Build history of the part. All positions in model axes, mm. A direction names the side the tool comes from. Give positions to 0.01 mm unless a question says otherwise; leave off trailing zeros. Order: outer loops, then holes, each group sorted by start corner. A loop starts at its lowest first (then second) coordinate and runs counter-clockwise, first axis right, second up. Notation, with made-up numbers: (62.25, -36.75) - (106.25, -36.75) arc R28 ccw to (106.25, -10.75) - close; hole circle Ø1 at (25.5, -10). An arc over 180 degrees is marked (long way). Answer in a Markdown table with one row per item.
```python
from build123d import *

# Parameters (mm, degrees)
BOSS_EXTRUDE1_DEPTH      = 13.97
BOSS_EXTRUDE1_DEPTH_BACK = 2.38125
SKETCH1_W                = 65.5
SKETCH1_H                = 47
SKETCH1_W_2              = 62.5
SKETCH1_H_2              = 44
SKETCH2_W                = 3.58
SKETCH2_H                = 3.58
BOSS_EXTRUDE2_DEPTH      = 13.97
SKETCH3_W                = 65.5
SKETCH3_H                = 47
SKETCH3_R                = 3.81
BOSS_EXTRUDE3_DEPTH      = 3
FILLET1_R                = 5
CUT_EXTRUDE1_DEPTH       = 1.5


with BuildPart() as part:
    # Sketch1 → Boss-Extrude1 (new, two sides: drawn at the far end of the back side and taken through both)
    with BuildSketch(Plane.XY.offset(-BOSS_EXTRUDE1_DEPTH_BACK)):
        with Locations((-101.75, -91.5)):
            Rectangle(SKETCH1_W, SKETCH1_H)
        with Locations((-101.75, -91.5)):
            Rectangle(SKETCH1_W_2, SKETCH1_H_2, mode=Mode.SUBTRACT)
    extrude(amount=BOSS_EXTRUDE1_DEPTH + BOSS_EXTRUDE1_DEPTH_BACK)

    # Sketch2 → Boss-Extrude2 (add)
    with BuildSketch(Plane.XY.offset(13.97)):
        with Locations((-131.21, -71.29)):
            Rectangle(SKETCH2_W, SKETCH2_H)
        with Locations((-131.21, -111.71)):
            Rectangle(SKETCH2_W, SKETCH2_H)
        with Locations((-72.29, -111.71)):
            Rectangle(SKETCH2_W, SKETCH2_H)
        with Locations((-72.29, -71.29)):
            Rectangle(SKETCH2_W, SKETCH2_H)
    extrude(amount=-BOSS_EXTRUDE2_DEPTH)

    # Sketch3 → Boss-Extrude3 (add)
    with BuildSketch(Plane.XY.offset(13.97)):
        with Locations((-101.75, -91.5)):
            Rectangle(SKETCH3_W, SKETCH3_H)
        with Locations((-105, -74.5)):
            Circle(SKETCH3_R, mode=Mode.SUBTRACT)
        with Locations((-90, -74.5)):
            Circle(SKETCH3_R, mode=Mode.SUBTRACT)
    extrude(amount=BOSS_EXTRUDE3_DEPTH)

    # Fillet1
    # the kernel refuses this fillet: 5 mm, written as the material it takes off along each edge
    with BuildSketch(Plane(origin=(-56.5, -68, 16.97), x_dir=(0, -1, 0), z_dir=(-1, 0, 0))) as fillet1_piece_1:
        with BuildLine():
            CenterArc((FILLET1_R, -FILLET1_R), FILLET1_R, 90, 90)
            Line((0, -FILLET1_R), (0, 0))
            Line((0, 0), (FILLET1_R, 0))
        make_face()
    extrude(amount=90.5, mode=Mode.SUBTRACT)
    with BuildSketch(Plane(origin=(-134.5, -55.5, 16.97), x_dir=(0, 0, -1), z_dir=(0, -1, 0)), Plane(origin=(-69, -127.5, 16.97), x_dir=(0, 0, -1), z_dir=(0, 1, 0))) as fillet1_piece_2:
        with BuildLine():
            CenterArc((FILLET1_R, FILLET1_R), FILLET1_R, 180, 90)
            Line((0, FILLET1_R), (0, 0))
            Line((0, 0), (FILLET1_R, 0))
        make_face()
    extrude(amount=72, mode=Mode.SUBTRACT)
    with BuildSketch(Plane(origin=(-147, -115, 16.97), x_dir=(0, 0, -1), z_dir=(1, 0, 0))) as fillet1_piece_3:
        with BuildLine():
            CenterArc((FILLET1_R, FILLET1_R), FILLET1_R, 180, 90)
            Line((0, FILLET1_R), (0, 0))
            Line((0, 0), (FILLET1_R, 0))
        make_face()
    extrude(amount=90.5, mode=Mode.SUBTRACT)

    # Sketch4 → Cut-Extrude1 (cut)
    with BuildSketch(Plane(origin=(-69, 0, 0), x_dir=(0, 0, -1), z_dir=(1, 0, 0))):
        with BuildLine():
            ThreePointArc((-10.276157649, -82.847028828), (-9.104584774, -80.018601703), (-6.276157649, -78.847028828))
            Line((-6.276157649, -78.847028828), (-2.784881052, -78.847028828))
            ThreePointArc((-2.784881052, -78.847028828), (0.043546073, -80.018601703), (1.215118948, -82.847028828))
            Line((1.215118948, -82.847028828), (1.215118948, -94.351328143))
            ThreePointArc((1.215118948, -94.351328143), (0.043546073, -97.179755268), (-2.784881052, -98.351328143))
            Line((-2.784881052, -98.351328143), (-6.276157649, -98.351328143))
            ThreePointArc((-6.276157649, -98.351328143), (-9.104584774, -97.179755268), (-10.276157649, -94.351328143))
            Line((-10.276157649, -94.351328143), (-10.276157649, -82.847028828))
        make_face()
    extrude(amount=-CUT_EXTRUDE1_DEPTH, mode=Mode.SUBTRACT)


solid = part.part
```
1. Cut at A-A on y = -90.5. Write the cut outline in (x, z).
Check result:
| item | result |
|---|---|
| outline | (-134.5, -2.38) - (-133, -2.38) - (-133, 13.97) - (-70.5, 13.97) - (-70.5, 10.28) - (-69, 10.28) - (-69, 11.97) arc R5 ccw to (-74, 16.97) - (-129.5, 16.97) arc R5 ccw to (-134.5, 11.97) - close; (-70.5, -2.38) - (-69, -2.38) - (-69, -1.22) - (-70.5, -1.22) - close |
2. Cut at B-B on y = -74.5. Write the cut outline in (x, z), and give its area (3 significant figures).
Check result:
| item | result |
|---|---|
| outline | (-134.5, -2.38) - (-133, -2.38) - (-133, 13.97) - (-108.81, 13.97) - (-108.81, 16.97) - (-129.5, 16.97) arc R5 ccw to (-134.5, 11.97) - close; (-101.19, 13.97) - (-93.81, 13.97) - (-93.81, 16.97) - (-101.19, 16.97) - close; (-86.19, 13.97) - (-70.5, 13.97) - (-70.5, -2.38) - (-69, -2.38) - (-69, 11.97) arc R5 ccw to (-74, 16.97) - (-86.19, 16.97) - close |
| area | 189 mm² |
3. Cut at D-D on x = -82. Write the cut outline in (y, z).
Check result:
| item | result |
|---|---|
| outline | (-115, -2.38) - (-113.5, -2.38) - (-113.5, 13.97) - (-69.5, 13.97) - (-69.5, -2.38) - (-68, -2.38) - (-68, 11.97) arc R5 ccw to (-73, 16.97) - (-110, 16.97) arc R5 ccw to (-115, 11.97) - close |
4. Cut at C-C on x = -89. Write the cut outline in (y, z), and give its area (3 significant figures).
Check result:
| item | result |
|---|---|
| outline | (-115, -2.38) - (-113.5, -2.38) - (-113.5, 13.97) - (-78.18, 13.97) - (-78.18, 16.97) - (-110, 16.97) arc R5 ccw to (-115, 11.97) - close; (-70.82, 13.97) - (-69.5, 13.97) - (-69.5, -2.38) - (-68, -2.38) - (-68, 11.97) arc R5 ccw to (-70.82, 16.47) - close |
| area | 158 mm² |
5. Two-plate mould, pull along X, no slides. Class faces 1 (the face through (-70.5, -92, 11)), 2 (the face through (-101.29, -69.5, 15.54)), 3 (the face through (-69, -97.1, 9.5)), 4 (the face through (-102, -113.5, 6)): +X half, -X half, draft (parallel to the pull), parting line (faces both ways), or undercut.
Check result:
| item | result |
|---|---|
| face 1 | undercut |
| face 2 | draft |
| face 3 | +X half |
| face 4 | undercut |
6. Which spindle directions (+Z, -Z, +X, -X, +Y, -Y) get a long thin tool onto all of the face, cutting with end or side? Do faces 5 (the face through (-102, -115, 5)), 6 (the face through (-74.08, -112, 7)), 7 (the face through (-70, -89, -1.215)). Say none if no direction does.
Check result:
| item | result |
|---|---|
| face 5 | +Z, -Z, +X, -X, -Y |
| face 6 | -Z |
| face 7 | +X |
7. Drop flat-ended pins along their axis: P1, Ø1.5, axis at x = -125, y = -75, coming from the -Z side; P2, Ø1, axis at x = -124, z = 13.5, coming from the -Y side; P3, Ø1.6, axis at x = -70, y = -90, coming from the +Z side. Give the stop position or say it passes through.
Check result:
| item | result |
|---|---|
| P1 | stops at z = 13.97 |
| P2 | stops at y = -114.89 |
| P3 | stops at z = 15.81 |
8. Probe line 1 (X direction, y = -78.5, z = 1); line 2 (X direction, y = -74.5, z = 15.3); line 3 (Y direction, x = -108, z = -0.75). List the from-to ranges inside material, lowest first.
Check result:
| item | result |
|---|---|
| line 1 | x = -134.5 to -133, -70.5 to -69 |
| line 2 | x = -133.23 to -108.81, -101.19 to -93.81, -86.19 to -70.27 |
| line 3 | y = -115 to -113.5, -69.5 to -68 |
